Could you check a few things on this model? Use its own coordinates, in mm. A direction names the side the tool comes from. Give positions to 0.01 mm unless a question says otherwise; leave off trailing zeros. Order: outer loops, then holes, each group sorted by start corner. A loop starts at its lowest first (then second) coordinate and runs counter-clockwise, first axis right, second up.
from build123d import *

# Parameters (mm, degrees)
F0_W        = 85.4306071997
F0_H        = 92.3714498058
F1_DEPTH    = 160.528
F2_T1_DEPTH = 692.3919824172
F3_T        = -2.54


# Not quite as in the source:
# - a fillet or chamfer that OpenCascade refuses, or shapes differently, is made with other operations: its cross-section is extruded or revolved along the edge and cut away or added


with BuildPart() as f1:
    # F0 (on Top) → F1 (new body)
    with BuildSketch(Plane.XY):
        with Locations((-126.2646093965, -30.766769778)):
            Rectangle(F0_W, F0_H)
    extrude(amount=F1_DEPTH)

    # F2: fillet of radius 127 on 1 edges, made by hand

    # F2_s2 → F2_t1 (cut)
    with BuildSketch(Plane.XZ.offset(-315.4292214306)):
        with BuildLine():
            ThreePointArc((-168.9799129963, 40.5238934777), (-145.4408062982, 114.1774307803), (-83.5493057966, 160.528))
            Line((-83.5493057966, 160.528), (-168.9799129963, 160.528))
            Line((-168.9799129963, 160.528), (-168.9799129963, 40.5238934777))
        make_face()
    extrude(amount=F2_T1_DEPTH, mode=Mode.SUBTRACT)

    # F3
    f3_openings = [f1.faces().sort_by_distance(p)[0] for p in [
        (-83.549306, -30.76677, 80.264),
    ]]
    offset(amount=F3_T, openings=f3_openings)


solid = f1.part
Item 1: Imagine slicing it at A-A on x = -145. List the corners of the cut face in (y, z) for me.
Findings:
outline: (-76.95, 0) - (15.42, 0) - (15.42, 114.79) - (-76.95, 114.79) - close; hole (-74.41, 2.54) - (12.88, 2.54) - (12.88, 110.36) - (-74.41, 110.36) - close
Item 2: We'd pull the mould along Z, two halves only. Please class faces 1 (the flat face through (-117, 15.419, 61)), 2 (the flat face through (-166.44, -31, 21)), 3 (the flat face through (-127, -30, 0)): +Z half, -Z half, draft (parallel to the pull), parting line (faces both ways), or undercut.
Findings:
face 1: draft
face 2: undercut
face 3: -Z half
Item 3: For faces 4 (the cylindrical face through (-144.24, -30.16, 111.47)), 5 (the flat face through (-83.549, 13.5, 79.9)), which set-ups out of +Z, -Z, +X, -X, +Y, -Y let a thin tool reach every point of the face, with its end or its side?
Findings:
face 4: +X
face 5: +Z, -Z, +X, +Y, -Y
Item 4: Please list where these lines run through material, in increasing order: line 1 along Y through (x, z) = (-92, 16.5); line 2 along X through (y, z) = (-10.5, 8); line 3 along Z through (x, y) = (-89.5, -6.5).
Findings:
line 1: y = -76.95 to -74.41, 12.88 to 15.42
line 2: x = -168.98 to -166.44
line 3: z = 0 to 2.54, 155.55 to 158.3
Item 5: For pin 1 (8 mm diameter, centred on x = -117.5, y = -33.5, fed in from +Z); pin 2 (8 mm diameter, centred on y = -11, z = 117, fed in from +X); pin 3 (6 mm diameter, centred on y = -35, z = 98, fed in from +X), each with a flat end and sliding along its axis, tell me the tip position at first contact or that it passes through.
Findings:
pin 1: stops at z = 145.47
pin 2: stops at x = -136.92
pin 3: stops at x = -150.76
Item 6: Imagine slicing it at D-D on x = -115. List the corners of the cut face in (y, z) for me.
Findings:
outline: (-76.95, 0) - (15.42, 0) - (15.42, 144.43) - (-76.95, 144.43) - close; hole (-74.41, 2.54) - (12.88, 2.54) - (12.88, 141.31) - (-74.41, 141.31) - close
Item 7: Imagine slicing it at B-B on z = 16.5. List the corners of the cut face in (x, y) for me.
Findings:
outline: (-168.98, -76.95) - (-83.55, -76.95) - (-83.55, -74.41) - (-166.44, -74.41) - (-166.44, 12.88) - (-83.55, 12.88) - (-83.55, 15.42) - (-168.98, 15.42) - close
Item 8: Imagine slicing it at C-C on y = -60. List the corners of the cut face in (x, z) for me, then the cut area to 4 significant figures.
Findings:
outline: (-168.98, 0) - (-83.55, 0) - (-83.55, 2.54) - (-166.44, 2.54) - (-166.44, 40.52) arc R124.46 cw to (-83.55, 157.84) - (-83.55, 160.53) arc R127 ccw to (-168.98, 40.52) - close
area: 707.5 mm2
